from build123d import *

# Parameters (mm, degrees)
SKETCH1_W           = 120
SKETCH1_H           = 20
BOSS_EXTRUDE1_DEPTH = 4
SKETCH2_R           = 3
CUT_EXTRUDE1_DEPTH  = 4
FILLET1_R           = 3


with BuildPart() as part:
    # Sketch1 → Boss-Extrude1 (new body)
    with BuildSketch(Plane(origin=(0, 0, 0), x_dir=(1, 0, 0), z_dir=(0, 1, 0))):
        Rectangle(SKETCH1_W, SKETCH1_H)
    extrude(amount=BOSS_EXTRUDE1_DEPTH)

    # Sketch2 → Cut-Extrude1 (cut)
    with BuildSketch(Plane(origin=(0, 4, 0), x_dir=(1, 0, 0), z_dir=(0, 1, 0))):
        with Locations((-50, 0)):
            Circle(SKETCH2_R)
        with Locations((50, 0)):
            Circle(SKETCH2_R)
    extrude(amount=-CUT_EXTRUDE1_DEPTH, mode=Mode.SUBTRACT)

    # Fillet1
    fillet1_edges = [part.edges().sort_by_distance(p)[0] for p in [
        (60, 2, 10),
        (-60, 2, 10),
        (-60, 2, -10),
        (60, 2, -10),
    ]]
    fillet(fillet1_edges, radius=FILLET1_R)


solid = part.part
Geometry: final body of the model. Coordinates: model frame, mm. Coordinates: 2 decimals unless noted, no trailing zeros. Loops run counter-clockwise (first coordinate to the right, second up) from the corner with the lowest first, then second, coordinate; pieces in that order, holes last. Notation, with made-up numbers: (49, -15) - (103, -15) arc R12 ccw to (103, -6) - close; hole circle Ø9 at (-34.5, 3.5). An arc over 180 degrees is marked (long way). One line per question, with ' | ' between items. Start each with the question number.
(1) Cut plane C-C on x = 50. Output: boundary loops of the cut face in (y, z).
(2) Cut plane B-B on y = 1.4. Output: boundary loops of the cut face in (x, z), and give its area (3 significant figures).
(3) Cut plane A-A on z = 0. Output: boundary loops of the cut face in (x, y).
(4) First-contact query: pin 1 (10 mm diameter, centred on x = 40.5, z = 1, fed in from -Y). Flat tip, straight axial feed; report the tip coordinate or a pass-through.
(5) Draft query along X for faces 1 (the flat face through (-1, 0, 0)), 2 (the cylindrical face through (-53, 2, 0)), 3 (the cylindrical face through (59.1, 2.03, -9.14)). Return one class per face: +X half, -X half, draft (parallel to the pull), parting line (faces both ways), or undercut.
(6) Ray query, L1, parallel to X at y = 2.25, z = 0; L2, parallel to Z at x = -50, y = 2.35; L3, parallel to X at y = 1.85, z = -2. Return the intervals inside material, ascending. Write a range as from..to.
Here are the results:
1) outline: (0, -10) - (4, -10) - (4, -3) - (0, -3) - close; (0, 3) - (4, 3) - (4, 10) - (0, 10) - close
2) outline: (-60, -7) arc R3 ccw to (-57, -10) - (57, -10) arc R3 ccw to (60, -7) - (60, 7) arc R3 ccw to (57, 10) - (-57, 10) arc R3 ccw to (-60, 7) - close; hole circle Ø6 at (-50, 0); hole circle Ø6 at (50, 0) | area: 2,340 mm²
3) outline: (-60, 0) - (-53, 0) - (-53, 4) - (-60, 4) - close; (-47, 0) - (47, 0) - (47, 4) - (-47, 4) - close; (53, 0) - (60, 0) - (60, 4) - (53, 4) - close
4) pin 1: y = 0
5) face 1: draft | face 2: undercut | face 3: +X half
6) L1: -60..-53, -47..47, 53..60 | L2: -10..-3, 3..10 | L3: -60..-52.24, -47.76..47.76, 52.24..60
